Model file for the job. Use its own axes, mm. Face numbers are marked on the shaded views. Round coordinates to 2 decimals unless told otherwise and drop trailing zeros. Loops run counter-clockwise (first coordinate to the right, second up) from the corner with the lowest first, then second, coordinate; pieces in that order, holes last. Notation, with made-up numbers: (-11, 26.25) - (41, 26.25) arc R26 ccw to (41, 53.25) - close; hole circle Ø11 at (87, 53.5). An arc over 180 degrees is marked (long way). Answer as a JSON object with one key per item and string values.
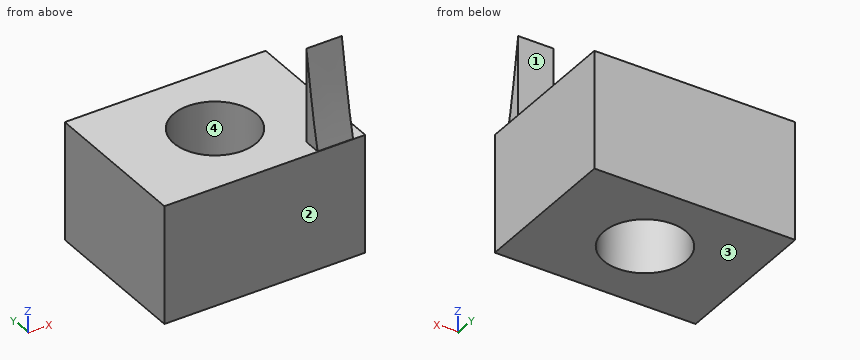
from build123d import *

# Parameters (mm, degrees)
SKETCH_W     = 17
SKETCH_H     = 13
SKETCH_R     = 3.5
PAD_DEPTH    = 10
PAD001_DEPTH = 3


with BuildPart() as obj1:
    # Sketch → Pad (new body)
    with BuildSketch(Plane.XY):
        Rectangle(SKETCH_W, SKETCH_H)
        Circle(SKETCH_R, mode=Mode.SUBTRACT)
    extrude(amount=PAD_DEPTH)


with BuildPart() as obj2:
    # Pad001 base: copy of obj1
    add(obj1.part)

    # Sketch003 → Pad001 (new body)
    with BuildSketch(Plane.YZ.offset(7.5)):
        with BuildLine():
            Line((4.98859, 17.9219), (4.98859, 9.858518))
            Line((4.98859, 9.858518), (6.5, 9.833834))
            add(Edge.make_bspline(
                [(4.98859, 17.9219), (5.5, 14.7982), (5.91318, 12.1235), (6.5, 9.833834)],
                knots=[0, 0, 0, 0, 1, 1, 1, 1], degree=3))
        make_face()
    pad001 = extrude(amount=-PAD001_DEPTH)


with BuildPart() as mirrored:
    # Mirrored base: copy of obj1
    add(obj1.part)

    # Mirrored: Pad001 across Sketch003 V_Axis
    add(pad001.mirror(Plane(origin=(7.5, 0, 0), x_dir=(1, 0, 0), z_dir=(0, 1, 0))))


solid = mirrored.part
1) Probe probe 1 along Y at (x, z) = (0, 7.25); probe 2 along Z at (x, y) = (4.75, 2.5); probe 3 along X at (y, z) = (-2.5, 5.5). List the from-to ranges inside material, lowest first.
Values follow:
{"probe 1": "-6.5 to -3.5, 3.5 to 6.5", "probe 2": "0 to 10", "probe 3": "-8.5 to -2.45, 2.45 to 8.5"}
2) Slice it at A-A on y = 0. List the corners of the cut face in (x, z).
Values follow:
{"outline": "(-8.5, 0) - (-3.5, 0) - (-3.5, 10) - (-8.5, 10) - close; (3.5, 0) - (8.5, 0) - (8.5, 10) - (3.5, 10) - close"}
3) Drop flat-ended pins along their axis: P1, Ø3.5, axis at x = 6, z = 14, coming from the +Y side; P2, Ø6.5, axis at x = 1, y = 0, coming from the +Z side. Give the stop position or say it passes through.
Values follow:
{"P1": "y = -4.99", "P2": "z = 10"}
4) Slice it at C-C on z = 8.75. List the corners of the cut face in (x, y), then the cut area to 3 significant figures.
Values follow:
{"outline": "(-8.5, -6.5) - (8.5, -6.5) - (8.5, 6.5) - (-8.5, 6.5) - close; hole circle Ø7 at (0, 0)", "area": "183 mm²"}
5) Slice it at D-D on x = -7. List the corners of the cut face in (y, z).
Values follow:
{"outline": "(-6.5, 0) - (6.5, 0) - (6.5, 10) - (-6.5, 10) - close"}
6) Slice it at B-B on x = 1. List the corners of the cut face in (y, z), then the cut area to 3 significant figures.
Values follow:
{"outline": "(-6.5, 0) - (-3.35, 0) - (-3.35, 10) - (-6.5, 10) - close; (3.35, 0) - (6.5, 0) - (6.5, 10) - (3.35, 10) - close", "area": "62.9 mm²"}
7) Two-plate mould, pull along Y, no slides. Class the marked faces 1, 2, 3 and 4: pulls with the +Y half, pulls with the -Y half, needs draft (parallel to the pull), parting line crosses it, or undercut.
Values follow:
{"face 1": "pulls with the +Y half", "face 2": "pulls with the -Y half", "face 3": "needs draft", "face 4": "undercut"}
